The listing builds one solid part. Answer for the finished solid, in the listing's coordinates (mm). A direction names the side the tool comes from. Coordinates: 2 decimals unless noted, no trailing zeros. Loops run counter-clockwise (first coordinate to the right, second up) from the corner with the lowest first, then second, coordinate; pieces in that order, holes last. Notation, with made-up numbers: M -18.5,-37 L 5.5,-37 A27 ccw 5.5,-16 Z; hole C 76.25,6 d10. An arc over 180 degrees is marked long. Answer as a JSON object with one key per item and string values. Group by question number.
1. Straight lines are drawn through the part: L1, parallel to X at y = -40.5, z = -5.5 (3 decimals); L2, parallel to Z at x = 20, y = -34 (3 decimals); L3, parallel to Y at x = 23.5, z = 16.5. For each, find the intervals that lie inside material, in ascending order.
2. A cutting plane is placed at C-C on y = -17. Give the vertices of the cut face in (x, z) (3 decimals), and give its area (3 significant figures).
3. A cutting plane is placed at A-A on y = -55.5. Give the vertices of the cut face in (x, z) (3 decimals), and give its area (3 significant figures).
4. A cutting plane is placed at B-B on x = 85. Give the vertices of the cut face in (y, z).
5. Given pin 1 (15 mm diameter, centred on x = 96.5, y = 4, fed in from -Z); pin 2 (15.5 mm diameter, centred on x = 49, z = 39.5, fed in from -Y); pin 3 (15.5 mm diameter, centred on x = 41.5, z = 31, fed in from +Y), each flat-ended and moving along its own axis, determine where each tip first touches the part or whether it passes through.
6. For faces 1 (the face through (22.225, -17, 18)), 2 (the face through (58, 0, 61.925)), 3 (the face through (32.73, 16.55, 51.97)), determine the directions among +Z, -Z, +X, -X, +Y, -Y from which every point of the face is accessible in a straight line to the end or side of a thin tool.
7. Determine the mould class of faces 4 (the face through (-39.8, -62, -0.1)), 5 (the face through (-2, -7.938, 31)), 6 (the face through (45.8, -0.4, 38.1)) for opening direction X: released by +X, released by -X, zero draft, split by the parting line, or undercut.
from build123d import *

# Parameters (mm, degrees)
F1_DEPTH = 63.5
F0_W     = 18.3103905071
F0_H     = 19.05
F2_DEPTH = 25.4
F3_DEPTH = 7.9375
F0_W_2   = 25.4
F0_H_2   = 28.575
F5_R     = 5.08


# Not quite as in the source:
# - a feature names something its author has since deleted; it is built from what else it names


with BuildPart() as f1:
    # F0 (on Front) → F1 (new body, symmetric)
    with BuildSketch(Plane.XZ):
        Polygon((-41.275, -9.525), (41.275, -9.525), (41.275, 9.525), (22.225, 9.525), (-41.275, 9.525), align=None)
    extrude(amount=F1_DEPTH, both=True)

    # F0 (on Front) → F2 (join, symmetric)
    with BuildSketch(Plane.XZ):
        with BuildLine():
            Line((22.225, 9.525), (41.275, 9.525))
            Line((41.275, 9.525), (41.275, 27.0002))
            ThreePointArc((41.275, 27.0002), (45.9246798487, 38.2255201513), (57.15, 42.8752))
            Line((57.15, 42.8752), (60.325, 42.8752))
            Line((60.325, 42.8752), (60.325, 61.9252))
            Line((60.325, 61.9252), (57.15, 61.9252))
            ThreePointArc((57.15, 61.9252), (32.4542956671, 51.6959043329), (22.225, 27.0002))
            Line((22.225, 27.0002), (22.225, 9.525))
        make_face()
        with Locations((69.4801952536, 52.4002)):
            Rectangle(F0_W, F0_H)
    extrude(amount=F2_DEPTH, both=True)

    # F0 (on Front) → F3 (join, symmetric)
    with BuildSketch(Plane.XZ):
        with BuildLine():
            add(Edge.make_bspline(
                [(-41.275, 9.525), (-33.2450978458, 46.1078099906), (9.6913008019, 63.8398453593), (57.15, 61.9252)],
                knots=[0, 0, 0, 0, 111.5045361635, 111.5045361635, 111.5045361635, 111.5045361635], degree=3))
            Line((-41.275, 9.525), (22.225, 9.525))
            Line((22.225, 9.525), (22.225, 27.0002))
            ThreePointArc((22.225, 27.0002), (32.4542956671, 51.6959043329), (57.15, 61.9252))
        make_face()
    extrude(amount=F3_DEPTH, both=True)

    # F0 (on Front) → F4 (revolve)
    with BuildSketch(Plane.XZ):
        with Locations((98.425, 52.4808056653)):
            Rectangle(F0_W_2, F0_H_2)
    revolve(axis=Axis((85.725, 0, 52.4808056653), (0, 0, 1)))

    # F5
    f5_edges = [f1.edges().sort_by_distance(p)[0] for p in [
        (41.275, -63.5, 0),
        (41.275, 63.5, 0),
        (-41.275, 63.5, 0),
        (-41.275, -63.5, 0),
    ]]
    fillet(f5_edges, radius=F5_R)


solid = f1.part
From the geometry:
{
 "1": {"L1": "x = -41.275 to 41.275", "L2": "z = -9.525 to 9.525", "L3": "y = -25.4 to 25.4"},
 "2": {"outline": "M -41.275,-9.525 L 41.275,-9.525 L 41.275,27 A15.875 cw 57.15,42.875 L 66.853,42.875 L 66.853,38.193 L 104.597,38.193 L 104.597,66.768 L 66.853,66.768 L 66.853,61.925 L 57.15,61.925 A34.925 ccw 22.225,27 L 22.225,9.525 L -41.275,9.525 Z", "area": "3,930 mm²"},
 "3": {"outline": "M -41.275,-9.525 L 41.275,-9.525 L 41.275,9.525 L -41.275,9.525 Z", "area": "1,570 mm²"},
 "4": {"outline": "M -25.39,38.19 L 25.39,38.19 L 25.39,66.77 L -25.39,66.77 Z"},
 "5": {"pin 1": "stops at z = 38.19", "pin 2": "stops at y = -25.4", "pin 3": "stops at y = 25.4"},
 "6": {"face 1": "+Z, -X, -Y", "face 2": "+Z", "face 3": "+Z, -X, +Y"},
 "7": {"face 4": "released by -X", "face 5": "zero draft", "face 6": "undercut"}
}
